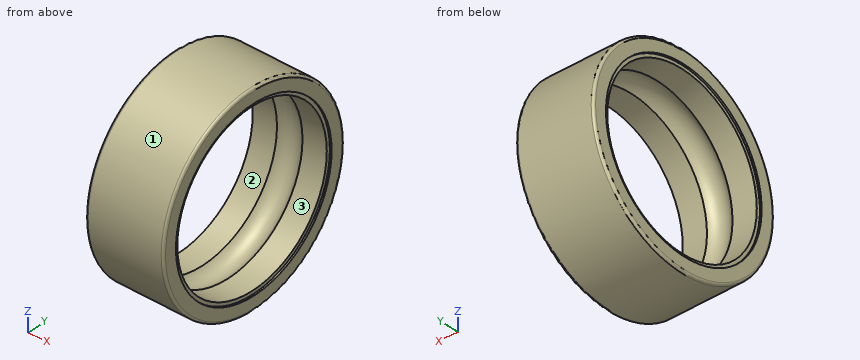
Autodesk Inventor part; units mm, degrees
ref_plane "mss_or_XY" through (0, 0, 0) normal (1, 0, 0) x (0, 0, -1)
ref_plane "mss_or_YZ" through (0, 0, 0) normal (0, 0, -1) x (0, 1, 0)
ref_plane "mss_or_ZX" through (0, 0, 0) normal (0, 1, 0) x (1, 0, 0)
sketch "Sketch_3" plane through (0, 0, 0) normal (0, 0, 1) x (1, 0, 0)
  line L0 (5, 0) -> (0, 0)
  line L1 (0, 5.604) -> (0.1125, 5.604)
  line L2 (0.1125, 5.604) -> (0.1125, 5.38)
  line L3 (0.1125, 5.38) -> (1.6776, 5.38)
  arc A0 (3.3224, 5.38) -> (1.6776, 5.38) centre (2.5, 4.75) ccw
  line L4 (3.3224, 5.38) -> (4.8875, 5.38)
  line L5 (4.8875, 5.38) -> (4.8875, 5.604)
  line L6 (4.8875, 5.604) -> (5, 5.604)
  line L7 (5, 5.604) -> (5, 6.35)
  arc A1 (5, 6.35) -> (4.85, 6.5) centre (4.85, 6.35) ccw
  line L8 (4.85, 6.5) -> (0.15, 6.5)
  arc A2 (0.15, 6.5) -> (0, 6.35) centre (0.15, 6.35) ccw
  line L9 (0, 6.35) -> (0, 5.604)
revolve "Revolution1" add sketch "Sketch_3" angle 360 about axis through (5, 0, 0) along (1, 0, 0)
ref_plane "mss_or_XY" through (0, 0, 0) normal (1, 0, 0) x (0, 0, -1)
ref_plane "mss_or_YZ" through (0, 0, 0) normal (0, 0, -1) x (0, 1, 0)
ref_plane "mss_or_ZX" through (0, 0, 0) normal (0, 1, 0) x (1, 0, 0)
ref_plane "mss_or11_XY" through (5, 0, 0) normal (1, 0, 0) x (0, 0, -1)
ref_plane "mss_or11_YZ" through (5, 0, 0) normal (0, 0, -1) x (0, 1, 0)
ref_plane "mss_or11_ZX" through (5, 0, 0) normal (0, 1, 0) x (1, 0, 0)
ref_plane "mss_or2_1_XY" through (1.75, 4.75, 0) normal (1, 0, 0) x (0, 0, -1)
ref_plane "mss_or2_1_YZ" through (1.75, 4.75, 0) normal (0, 0, -1) x (0, 1, 0)
ref_plane "mss_or2_1_ZX" through (1.75, 4.75, 0) normal (0, 1, 0) x (1, 0, 0)
ref_plane "mss_or2_2_XY" through (1.75, 3.3588, 3.3588) normal (1, 0, 0) x (0, 0, -1)
ref_plane "mss_or2_2_YZ" through (1.75, 3.3588, 3.3588) normal (0, 0, -1) x (0, 1, 0)
ref_plane "mss_or2_2_ZX" through (1.75, 3.3588, 3.3588) normal (0, 1, 0) x (1, 0, 0)
ref_plane "mss_or2_3_XY" through (1.75, 0, 4.75) normal (1, 0, 0) x (0, 0, -1)
ref_plane "mss_or2_3_YZ" through (1.75, 0, 4.75) normal (0, 0, -1) x (0, 1, 0)
ref_plane "mss_or2_3_ZX" through (1.75, 0, 4.75) normal (0, 1, 0) x (1, 0, 0)
ref_plane "mss_or2_4_XY" through (1.75, -3.3588, 3.3588) normal (1, 0, 0) x (0, 0, -1)
ref_plane "mss_or2_4_YZ" through (1.75, -3.3588, 3.3588) normal (0, 0, -1) x (0, 1, 0)
ref_plane "mss_or2_4_ZX" through (1.75, -3.3588, 3.3588) normal (0, 1, 0) x (1, 0, 0)
ref_plane "mss_or2_5_XY" through (1.75, -4.75, 0) normal (1, 0, 0) x (0, 0, -1)
ref_plane "mss_or2_5_YZ" through (1.75, -4.75, 0) normal (0, 0, -1) x (0, 1, 0)
ref_plane "mss_or2_5_ZX" through (1.75, -4.75, 0) normal (0, 1, 0) x (1, 0, 0)
ref_plane "mss_or2_6_XY" through (1.75, -3.3588, -3.3588) normal (1, 0, 0) x (0, 0, -1)
ref_plane "mss_or2_6_YZ" through (1.75, -3.3588, -3.3588) normal (0, 0, -1) x (0, 1, 0)
ref_plane "mss_or2_6_ZX" through (1.75, -3.3588, -3.3588) normal (0, 1, 0) x (1, 0, 0)
ref_plane "mss_or2_7_XY" through (1.75, 0, -4.75) normal (1, 0, 0) x (0, 0, -1)
ref_plane "mss_or2_7_YZ" through (1.75, 0, -4.75) normal (0, 0, -1) x (0, 1, 0)
ref_plane "mss_or2_7_ZX" through (1.75, 0, -4.75) normal (0, 1, 0) x (1, 0, 0)
ref_plane "mss_or2_8_XY" through (1.75, 3.3588, -3.3588) normal (1, 0, 0) x (0, 0, -1)
ref_plane "mss_or2_8_YZ" through (1.75, 3.3588, -3.3588) normal (0, 0, -1) x (0, 1, 0)
ref_plane "mss_or2_8_ZX" through (1.75, 3.3588, -3.3588) normal (0, 1, 0) x (1, 0, 0)
ref_plane "mss_or21_1_XY" through (2.5, 4.75, 0) normal (1, 0, 0) x (0, 0, -1)
ref_plane "mss_or21_1_YZ" through (2.5, 4.75, 0) normal (0, 0, -1) x (0, 1, 0)
ref_plane "mss_or21_1_ZX" through (2.5, 4.75, 0) normal (0, 1, 0) x (1, 0, 0)
ref_plane "mss_or21_2_XY" through (2.5, 3.3588, 3.3588) normal (1, 0, 0) x (0, 0, -1)
ref_plane "mss_or21_2_YZ" through (2.5, 3.3588, 3.3588) normal (0, 0, -1) x (0, 1, 0)
ref_plane "mss_or21_2_ZX" through (2.5, 3.3588, 3.3588) normal (0, 1, 0) x (1, 0, 0)
ref_plane "mss_or21_3_XY" through (2.5, 0, 4.75) normal (1, 0, 0) x (0, 0, -1)
ref_plane "mss_or21_3_YZ" through (2.5, 0, 4.75) normal (0, 0, -1) x (0, 1, 0)
ref_plane "mss_or21_3_ZX" through (2.5, 0, 4.75) normal (0, 1, 0) x (1, 0, 0)
ref_plane "mss_or21_4_XY" through (2.5, -3.3588, 3.3588) normal (1, 0, 0) x (0, 0, -1)
ref_plane "mss_or21_4_YZ" through (2.5, -3.3588, 3.3588) normal (0, 0, -1) x (0, 1, 0)
ref_plane "mss_or21_4_ZX" through (2.5, -3.3588, 3.3588) normal (0, 1, 0) x (1, 0, 0)
ref_plane "mss_or21_5_XY" through (2.5, -4.75, 0) normal (1, 0, 0) x (0, 0, -1)
ref_plane "mss_or21_5_YZ" through (2.5, -4.75, 0) normal (0, 0, -1) x (0, 1, 0)
ref_plane "mss_or21_5_ZX" through (2.5, -4.75, 0) normal (0, 1, 0) x (1, 0, 0)
ref_plane "mss_or21_6_XY" through (2.5, -3.3588, -3.3588) normal (1, 0, 0) x (0, 0, -1)
ref_plane "mss_or21_6_YZ" through (2.5, -3.3588, -3.3588) normal (0, 0, -1) x (0, 1, 0)
ref_plane "mss_or21_6_ZX" through (2.5, -3.3588, -3.3588) normal (0, 1, 0) x (1, 0, 0)
ref_plane "mss_or21_7_XY" through (2.5, 0, -4.75) normal (1, 0, 0) x (0, 0, -1)
ref_plane "mss_or21_7_YZ" through (2.5, 0, -4.75) normal (0, 0, -1) x (0, 1, 0)
ref_plane "mss_or21_7_ZX" through (2.5, 0, -4.75) normal (0, 1, 0) x (1, 0, 0)
ref_plane "mss_or21_8_XY" through (2.5, 3.3588, -3.3588) normal (1, 0, 0) x (0, 0, -1)
ref_plane "mss_or21_8_YZ" through (2.5, 3.3588, -3.3588) normal (0, 0, -1) x (0, 1, 0)
ref_plane "mss_or21_8_ZX" through (2.5, 3.3588, -3.3588) normal (0, 1, 0) x (1, 0, 0)
properties part number "W686ZZ Outer ring"
CAD build for the part. Positions are in the model's coordinates, mm. Face numbers are marked on the shaded views. Give positions to 0.01 mm unless a question says otherwise; leave off trailing zeros. Order: outer loops, then holes, each group sorted by start corner. A loop starts at its lowest first (then second) coordinate and runs counter-clockwise, first axis right, second up.
(1) Saw through at A-A, the plane z = 0. Give the cut face in (x, y), then the cut area to 3 significant figures.
(2) Saw through at D-D, the plane x = 3.15. Give the cut face in (y, z).
(3) Mould opens along Y. For the marked faces 1, 2 and 3 say: released by +Y, released by -Y, zero draft, split by the parting line, or undercut.
(4) Saw through at C-C, the plane x = 4.4. Give the cut face in (y, z).
(5) Flat gauge pins, fed straight in: pin 1 (6.5 mm diameter, centred on y = 0, z = 0, fed in from -X) (1 decimal); pin 2 (3 mm diameter, centred on y = -1.5, z = 4.5, fed in from -X); pin 3 (1.5 mm diameter, centred on x = 3, z = 1, fed in from -Y). Where does each tip first touch, or does it go through?
(6) Drill centre lines: L1, parallel to Z at x = 1.1, y = 0; L2, parallel to Z at x = 2.65, y = 1.5; L3, parallel to Y at x = 4.7, z = -4.75. Where is each one in solid material? Low to high.
Results found:
1. outline: (0, -6.35) arc R0.15 ccw to (0.15, -6.5) - (4.85, -6.5) arc R0.15 ccw to (5, -6.35) - (5, -5.6) - (4.89, -5.6) - (4.89, -5.38) - (3.32, -5.38) arc R1.04 cw to (1.68, -5.38) - (0.11, -5.38) - (0.11, -5.6) - (0, -5.6) - close; (0, 5.6) - (0.11, 5.6) - (0.11, 5.38) - (1.68, 5.38) arc R1.04 cw to (3.32, 5.38) - (4.89, 5.38) - (4.89, 5.6) - (5, 5.6) - (5, 6.35) arc R0.15 ccw to (4.85, 6.5) - (0.15, 6.5) arc R0.15 ccw to (0, 6.35) - close
1. area: 10.1 mm2
2. outline: circle Ø13 at (0, 0); hole circle Ø11.11 at (0, 0)
3. face 1: split by the parting line
3. face 2: undercut
3. face 3: undercut
4. outline: circle Ø13 at (0, 0); hole circle Ø10.76 at (0, 0)
5. pin 1: passes through
5. pin 2: stops at x = 0
5. pin 3: stops at y = -6.5
6. L1: z = -6.5 to -5.38, 5.38 to 6.5
6. L2: z = -6.32 to -5.58, 5.58 to 6.32
6. L3: y = -4.44 to -2.53, 2.53 to 4.44
